The listing builds one solid part. Answer for the finished solid, in the listing's coordinates (mm). Face numbers are marked on the shaded views. Round coordinates to 2 decimals unless told otherwise and drop trailing zeros. Write each loop counter-clockwise with the first axis right and the second up, starting at its lowest first coordinate (ties: lowest second). Pieces come first, ordered by that corner, then holes. Notation, with made-up numbers: M 43.5,67.5 L 84.5,67.5 A23 ccw 84.5,95.5 Z; hole C -15.75,-34.75 d2. An arc over 180 degrees is marked long. Write each question's results on one line, items separated by ' | '.
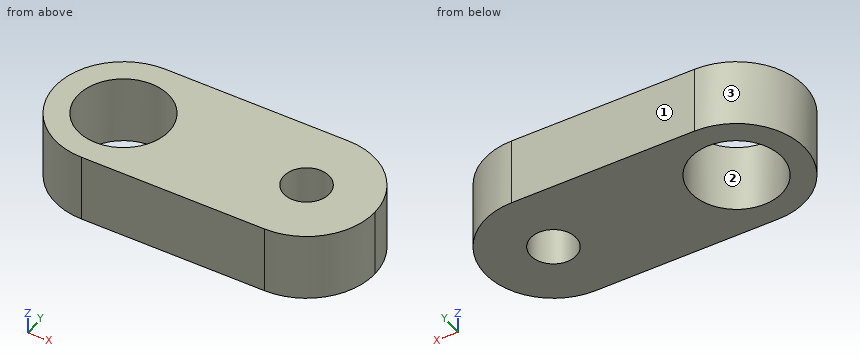
from build123d import *

# Parameters (mm, degrees)
SKETCH_1_R      = 2
SKETCH_1_R_2    = 1
EXTRUDE_1_DEPTH = 3


with BuildPart() as part:
    # Эскиз1 → Бобышка-Вытянуть1 (new body)
    with BuildSketch(Plane.XY):
        with BuildLine():
            Line((0, 3), (8, 3))
            ThreePointArc((8, 3), (10.121320344, 2.121320344), (11, 0))
            ThreePointArc((11, 0), (10.121320344, -2.121320344), (8, -3))
            Line((8, -3), (0, -3))
            ThreePointArc((0, -3), (-3, 0), (0, 3))
        make_face()
        Circle(SKETCH_1_R, mode=Mode.SUBTRACT)
        with Locations((8, 0)):
            Circle(SKETCH_1_R_2, mode=Mode.SUBTRACT)
    extrude(amount=EXTRUDE_1_DEPTH)


solid = part.part
1) Each of these flat-tipped pins is pushed along its axis until it touches: pin 1 (1.5 mm diameter, centred on x = -1.5, z = 1, fed in from -Y); pin 2 (1.5 mm diameter, centred on y = -1, z = 1, fed in from +X). Where does it stop, or does it pass through?
Return value:
pin 1: y = -2.9 | pin 2: x = 10.99
2) Section B-B (x = 7.75) is taken. Determine the outline of the cut face in (y, z).
Return value:
outline: M -3,0 L -0.97,0 L -0.97,3 L -3,3 Z; M 0.97,0 L 3,0 L 3,3 L 0.97,3 Z
3) Section D-D (x = -0.75) is taken. Determine the outline of the cut face in (y, z).
Return value:
outline: M -2.9,0 L -1.85,0 L -1.85,3 L -2.9,3 Z; M 1.85,0 L 2.9,0 L 2.9,3 L 1.85,3 Z
4) Section C-C (y = 0.25) is taken. Determine the outline of the cut face in (x, z), then the cut area to 3 significant figures.
Return value:
outline: M -2.99,0 L -1.98,0 L -1.98,3 L -2.99,3 Z; M 1.98,0 L 7.03,0 L 7.03,3 L 1.98,3 Z; M 8.97,0 L 10.99,0 L 10.99,3 L 8.97,3 Z | area: 24.2 mm²
5) The mould has two halves that part along X. Classify the marked faces 1, 2 and 3: +X half, -X half, draft (parallel to the pull), parting line (faces both ways), or undercut.
Return value:
face 1: draft | face 2: undercut | face 3: -X half
6) Section A-A (z = 2.8) is taken. Determine the outline of the cut face in (x, y), then the cut area to 3 significant figures.
Return value:
outline: M 0,-3 L 8,-3 A3 ccw 8,3 L 0,3 A3 ccw Z; hole C 0,0 d4; hole C 8,0 d2 | area: 60.6 mm²
7) Find the intervals of material crossed by line 1 (Y direction, x = 0, z = 0.7); line 2 (X direction, y = 0.75, z = 1.8); line 3 (X direction, y = -0.5, z = 1.8), in increasing order.
Return value:
line 1: -3 to -2, 2 to 3 | line 2: -2.9 to -1.85, 1.85 to 7.34, 8.66 to 10.9 | line 3: -2.96 to -1.94, 1.94 to 7.13, 8.87 to 10.96
